Check sheet for the modelled part. Datum: model origin and axes. Units: mm. A direction names the side the tool comes from. Coordinates: 2 decimals unless noted, no trailing zeros. Order: outer loops, then holes, each group sorted by start corner. A loop starts at its lowest first (then second) coordinate and runs counter-clockwise, first axis right, second up. Notation, with made-up numbers: M 0.5,-40 L 40.5,-40 A19 ccw 40.5,-25 Z; hole C 63.5,3.25 d10. An arc over 180 degrees is marked long. Answer in a Markdown table with one row per item. Add a question column.
Autodesk Inventor part; units mm, degrees
ref_plane "Work Plane5" through (0, -16.5, 0) normal (0, -1, 0) x (1, 0, 0)
ref_plane "YZ Plane" through (0, 0, 0) normal (1, 0, 0) x (0, 1, 0)
ref_plane "XZ Plane" through (0, 0, 0) normal (0, 1, 0) x (-1, 0, 0)
sketch "Sketch1" plane through (0, 0, 0) normal (0, 0, 1) x (1, 0, 0)
  line L0 (0, 19.9282) -> (4, 13)
  line L1 (4, 13) -> (4, -14)
  line L2 (4, -14) -> (0, -14)
  line L3 (0, -25.9015) -> (0, 19.9282)
  line L4 (2.75, -12.5) -> (-2.75, -12.5)
  line L5 (-2.75, -12.5) -> (-2.75, 12.5)
  line L6 (-2.75, 12.5) -> (2.75, 12.5)
  line L7 (2.75, 12.5) -> (2.75, -12.5)
  point P0 (0, 0)
  dimension "d0" = 30
  dimension "d1" = 4
  dimension "d45" = 14
  dimension "d47" = 2.75
  dimension "d48" = 13
  dimension "d81" = 12.5
  dimension "d82" = 12.5
revolve "main cylinder" add sketch "Sketch1" angle 360 about axis through (0, -25.9015, 0) along (0, 1, 0) contours L0 L1 L2 L3 L4 L7 L6 | L6 L7 L4 L3
extrude "main window" cut sketch "Sketch1" against normal mid plane 25.4 contours L6 L7 L4 L3 | L3 L4 L5 L6
sketch "Sketch2" plane through (-2.75, -12.5, 2.9047) normal (1, 0, 0) x (0, 0, -1)
  point P0 (2.9047, 12.5)
  point P1 (2.9047, 12.5)
hole "full side hole" at (-2.75, 0, 0) direction (-1, 0, 0) diameter 1 depth 25.4
sketch "Sketch3" plane through (0, -14, 0) normal (0, -1, 0) x (1, 0, 0)
  circle A0 centre (0, 0) radius 4
  line L0 (-3.9686, 0.5) -> (-3.5, 0.5)
  line L1 (-3.5, 0.5) -> (-3.5, -0.5)
  line L2 (-3.5, -0.5) -> (-3.9686, -0.5)
  line L3 (-10.1288, 0) -> (5.4225, 0)
  line L4 (0, 8.0973) -> (0, -8.0973)
  line L5 (-2.9513, 2.7) -> (2.9513, 2.7)
  line L6 (3.9686, 0.5) -> (3.5, 0.5)
  line L7 (3.5, 0.5) -> (3.5, -0.5)
  line L8 (3.5, -0.5) -> (3.9686, -0.5)
  line L9 (-1.75, 2.7) -> (-1.7428, 2.7) construction
  line L10 (1.7428, 1.7526) -> (1.75, 1.7526)
  line L11 (-1.7428, 1.7526) -> (-1.75, 1.7526)
  line L12 (1.7428, 2.7) -> (1.75, 2.7) construction
  line L13 (-1.7428, 2.7) -> (1.7428, 2.7)
  point P0 (0, 0)
  point P1 (0, -3)
  point P2 (0, -7)
  point P3 (-3.5536, -1.8362)
  point P4 (3.5536, -1.8362)
  dimension "d14" = 1
  dimension "d15" = 3.5
  dimension "d20" = 3
  dimension "d35" = 2.7
  dimension "d38" = 7
hole "partial side hole" at (-2.75, 0, 0) direction (-1, 0, 0) diameter 2 depth 0.75
extrude "side channels" cut sketch "Sketch3" against normal blind 14.5 contours L3 L7 L6 A0 | A0 L8 L7 L3 | A0 L3 L1 L2 | L3 A0 L0 L1
hole "thread hole" at (0, -14, -3) direction (0, 1, 0) diameter 1 end through all
extrude "Extrusion4" cut sketch "Sketch3" against normal blind 10 contours L5 L4 A0 | L4 L5 A0
extrude "Extrusion5" cut sketch "Sketch3" along normal blind 20 contours A0 L3 L1 L2 | L3 A0 L0 L1
fillet "Fillet1" radius 2 4 edges at (-2.75, 12.5, 0) (2.75, 12.5, 0) (-2.75, -12.5, -0.1024) (2.75, -12.5, -0.1024)
mirror "Mirror4" about plane through (0, 0, 0) normal (1, 0, 0) of "partial side hole", "full side hole"
sketch "Sketch8" plane through (0, -14, 0) normal (0, -1, 0) x (1, 0, 0)
  line L0 (2.9513, 2.7) -> (-2.9513, 2.7)
  line L1 (2.9513, 2.7) -> (-2.9513, 2.7)
  arc A0 (-2.9513, 2.7) -> (-3.9686, 0.5) centre (0, 0) ccw
  line L2 (-3.9686, 0.5) -> (-3.5, 0.5)
  line L3 (-3.5, 0.5) -> (-3.5, -0.5)
  line L4 (-3.5, -0.5) -> (-3.9686, -0.5)
  arc A1 (-3.9686, -0.5) -> (3.9686, -0.5) centre (0, 0) ccw
  line L5 (3.9686, -0.5) -> (3.5, -0.5)
  line L6 (3.5, -0.5) -> (3.5, 0.5)
  line L7 (3.5, 0.5) -> (3.9686, 0.5)
  arc A2 (3.9686, 0.5) -> (2.9513, 2.7) centre (0, 0) ccw
  circle A3 centre (0, -3) radius 0.5
  line L8 (-2.9513, 2.7) -> (2.9513, 2.7)
  circle A4 centre (0, 0) radius 4
  line L9 (-2.4, -1) -> (-2.4, 2.7)
  line L10 (2.4, -1) -> (2.4, 2.7)
  line L11 (-2.4, -1) -> (2.4, -1)
  point P0 (0, 15.9155)
  point P1 (0, -1)
  dimension "d105" = 4.8
  dimension "d115" = 1
extrude "Extrusion11" add sketch "Sketch8" along normal blind 15 contours L10 L11 L9 L0
ref_plane "Work Plane5" through (0, -16.5, 0) normal (0, -1, 0) x (1, 0, 0)
sketch "Sketch9" plane through (0, -16.5, 0) normal (0, -1, 0) x (1, 0, 0)
  line L0 (2.4, -1) -> (-2.4, -1)
  line L1 (-2.4, -1) -> (-2.4, 2.7)
  line L2 (2.4, 2.7) -> (2.4, -1)
  line L3 (-2.9513, 2.7) -> (2.9513, 2.7)
  line L4 (2, 2.5) -> (-2, 2.5)
  line L5 (-2, 2.5) -> (-2, -0.8)
  line L6 (-2, -0.8) -> (2, -0.8)
  line L7 (2, -0.8) -> (2, 2.5)
  point P0 (0, 0)
  point P1 (0, 2.5)
  point P2 (0, -1)
  point P3 (0, -1)
  dimension "d108" = 4
  dimension "d109" = 3.3
  dimension "d111" = 0.2
  dimension "d112" = 0.4
extrude "Extrusion12" cut sketch "Sketch9" along normal blind 0.5
properties part number "Rotator Frame_xw" material "SAN Plastic"
1. Set-up check for faces 4 (the flat face through (3.5, 0.7, 0)), 5 (the flat face through (0, -15, -1)), 6 (the flat face through (-3.5, -8, 0)), 7 (the flat face through (3.5, -8, 0)), 8 (the cylindrical face through (-2.15, 11.93, 0.06)): record each of +Z, -Z, +X, -X, +Y, -Y from which the full face is reachable in a straight line by a thin tool's end or side.
2. Section check A-A on y = 0. Enter the section's corners in (x, z), then the cut area to 3 significant figures.
3. Release check for a two-part mould opening along Z. For faces 1 (the cylindrical face through (3, -1, 0)), 2 (the flat face through (-2.4, -23, 1)), 3 (the flat face through (0, -23, -1)) record: released by +Z, released by -Z, zero draft, split by the parting line, or undercut.
4. Section check B-B on y = -5.5. Enter the section's corners in (x, z), then the cut area to 3 significant figures.
5. Go/stop test with flat-tipped pins: pin 1 Ø3 at (y, z) = (-15, 1) entering from -X; pin 2 Ø0.5 at (x, y) = (3.5, -5.5) entering from -Z; pin 3 Ø4.5 at (y, z) = (-2, -1) entering from +X. Record where each tip stops, or that it passes through.
6. Scan lines: line 1 (Y direction, x = 3.2, z = 0); line 2 (X direction, y = -20, z = 0.5); line 3 (Z direction, x = -1.5, y = -22.5). Record each from-to range of solid material in increasing order.
7. Section check C-C on y = -22. Enter the section's corners in (x, z), then the cut area to 3 significant figures.
Result sheet:
| question | item | result |
|---|---|---|
| 1 | face 4 | none |
| 1 | face 5 | -Z, +X, -X, -Y |
| 1 | face 6 | -X, -Y |
| 1 | face 7 | +X, -Y |
| 1 | face 8 | +Z, -Z |
| 2 | outline | M -3.97,-0.5 A4 ccw -2.75,-2.9 L -2.75,-1 L -3.5,-1 L -3.5,-0.5 Z; M -3.97,0.5 L -3.5,0.5 L -3.5,1 L -2.75,1 L -2.75,2.9 A4 ccw Z; M 2.75,-2.9 A4 ccw 3.97,-0.5 L 3.5,-0.5 L 3.5,-1 L 2.75,-1 Z; M 2.75,1 L 3.5,1 L 3.5,0.5 L 3.97,0.5 A4 ccw 2.75,2.9 Z |
| 2 | area | 6.05 mm^2 |
| 3 | face 1 | undercut |
| 3 | face 2 | zero draft |
| 3 | face 3 | released by -Z |
| 4 | outline | M -3.97,-0.5 A4 ccw -2.75,-2.9 L -2.75,2.7 L -2.95,2.7 A4 ccw -3.97,0.5 L -3.5,0.5 L -3.5,-0.5 Z; M 2.75,-2.9 A4 ccw 3.97,-0.5 L 3.5,-0.5 L 3.5,0.5 L 3.97,0.5 A4 ccw 2.95,2.7 L 2.75,2.7 Z |
| 4 | area | 9.01 mm^2 |
| 5 | pin 1 | x = -3.97 |
| 5 | pin 2 | z = -2.33 |
| 5 | pin 3 | x = 3.97 |
| 6 | line 1 | -14 to -1, 1 to 14.39 |
| 6 | line 2 | -2.4 to 2.4 |
| 6 | line 3 | -1 to 2.7 |
| 7 | outline | M -2.4,-1 L 2.4,-1 L 2.4,2.7 L -2.4,2.7 Z |
| 7 | area | 17.8 mm^2 |
